```python
from build123d import *

# Parameters (mm, degrees)
ESTRUSIONE_ESTRUSIONE1_DEPTH      = 10
ESTRUSIONE_ESTRUSIONE1_DEPTH_BACK = 3
SCHIZZO1_W                        = 89
SCHIZZO1_H                        = 2
SCHIZZO2_W                        = 25
SCHIZZO2_H                        = 2
TAGLIO_ESTRUSIONE1_DEPTH          = 10
SCHIZZO3_W                        = 20
SCHIZZO3_H                        = 3
TAGLIO_ESTRUSIONE2_DEPTH          = 10
RACCORDO1_R                       = 8


with BuildPart() as part:
    # Schizzo1 → Estrusione-Estrusione1 (new, two sides: drawn at the far end of the back side and taken through both)
    with BuildSketch(Plane.XY.offset(-ESTRUSIONE_ESTRUSIONE1_DEPTH_BACK)):
        with Locations((0, 22.5)):
            Rectangle(SCHIZZO1_W, SCHIZZO1_H)
    extrude(amount=ESTRUSIONE_ESTRUSIONE1_DEPTH + ESTRUSIONE_ESTRUSIONE1_DEPTH_BACK)

    # Schizzo2 → Taglio-Estrusione1 (cut)
    with BuildSketch(Plane.XZ.offset(-21.5)):
        with Locations((-25, 6)):
            Rectangle(SCHIZZO2_W, SCHIZZO2_H)
        with Locations((25, 6)):
            Rectangle(SCHIZZO2_W, SCHIZZO2_H)
    extrude(amount=-TAGLIO_ESTRUSIONE1_DEPTH, mode=Mode.SUBTRACT)

    # Schizzo3 → Taglio-Estrusione2 (cut)
    with BuildSketch(Plane(origin=(0, 23.5, 0), x_dir=(1, 0, 0), z_dir=(0, 1, 0))):
        with Locations((0, 1.5)):
            Rectangle(SCHIZZO3_W, SCHIZZO3_H)
    extrude(amount=-TAGLIO_ESTRUSIONE2_DEPTH, mode=Mode.SUBTRACT)

    # Raccordo1
    raccordo1_edges = [part.edges().sort_by_distance(p)[0] for p in [
        (-44.5, 22.5, 10),
        (44.5, 22.5, 10),
    ]]
    fillet(raccordo1_edges, radius=RACCORDO1_R)


solid = part.part
```
Check sheet for the modelled part. Datum: model origin and axes. Units: mm. A direction names the side the tool comes from. Round coordinates to 2 decimals unless told otherwise and drop trailing zeros. Loops run counter-clockwise (first coordinate to the right, second up) from the corner with the lowest first, then second, coordinate; pieces in that order, holes last. Notation, with made-up numbers: (-10.5, 51.25) -> (41.5, 51.25) arc R25 ccw to (41.5, 63.25) -> close; hole circle Ø6 at (-3, 79). An arc over 180 degrees is marked (long way). Write item = value, one per line. Start each with the question number.
1) Release check for a two-part mould opening along X. For faces 4 (the flat face through (27, 23, -3)), 5 (the cylindrical face through (-42.219, 22.514, 7.594)), 6 (the flat face through (10, 23, -1)) record: released by +X, released by -X, zero draft, split by the parting line, or undercut.
2) Sectioned sample at C-C, the plane y = 22.15. Record the cut outline in (x, z), plus the area to 3 significant figures.
3) Sectioned sample at B-B, the plane z = -0.75. Record the cut outline in (x, y).
4) Gauge pin test, flat ends, axial feed: pin 1 Ø0.6 at (y, z) = (22.5, 6) entering from +X; pin 2 Ø1 at (y, z) = (22, 5.5) entering from -X; pin 3 Ø5 at (x, z) = (-18.5, 5.5) entering from -Y; pin 4 Ø1 at (y, z) = (22.5, 6.5) entering from -X. Record the tip position at first contact, or that the pin passes through.
5) Set-up check for faces 1 (the flat face through (0, 23, 0)), 2 (the flat face through (12.5, 22, 6)), 3 (the flat face through (-1, 23.5, 3)): record each of +Z, -Z, +X, -X, +Y, -Y from which the full face is reachable in a straight line by a thin tool's end or side.
6) Sectioned sample at A-A, the plane x = 19. Record the cut outline in (y, z), plus the area to 3 significant figures.
7) Sectioned sample at D-D, the plane x = 5. Record the cut outline in (y, z), plus the area to 3 significant figures.
8) Thickness scan on probe 1 along X at (y, z) = (21.7, -1.5); probe 2 along Z at (x, y) = (29, 22.4); probe 3 along X at (y, z) = (22, 6). Record the ranges inside material, lowest first.
Results are:
q1.face_4 = zero draft
q1.face_5 = released by -X
q1.face_6 = undercut
q2.outline = (-44.5, -3) -> (-10, -3) -> (-10, 0) -> (10, 0) -> (10, -3) -> (44.5, -3) -> (44.5, 2) arc R8 ccw to (36.5, 10) -> (-36.5, 10) arc R8 ccw to (-44.5, 2) -> close; hole (-37.5, 5) -> (-12.5, 5) -> (-12.5, 7) -> (-37.5, 7) -> close; hole (12.5, 5) -> (37.5, 5) -> (37.5, 7) -> (12.5, 7) -> close
q2.area = 970 mm^2
q3.outline = (-44.5, 21.5) -> (-10, 21.5) -> (-10, 23.5) -> (-44.5, 23.5) -> close; (10, 21.5) -> (44.5, 21.5) -> (44.5, 23.5) -> (10, 23.5) -> close
q4.pin_1 = 43.59
q4.pin_2 = -43.92
q4.pin_3 = 21.5
q4.pin_4 = -43.43
q5.face_1 = -Z, +Y, -Y
q5.face_2 = +Y, -Y
q5.face_3 = +Z, -Z, +X, -X, +Y
q6.outline = (21.5, -3) -> (23.5, -3) -> (23.5, 5) -> (21.5, 5) -> close; (21.5, 7) -> (23.5, 7) -> (23.5, 10) -> (21.5, 10) -> close
q6.area = 22.0 mm^2
q7.outline = (21.5, 0) -> (23.5, 0) -> (23.5, 10) -> (21.5, 10) -> close
q7.area = 20.0 mm^2
q8.probe_1 = -44.5 to -10, 10 to 44.5
q8.probe_2 = -3 to 5, 7 to 10
q8.probe_3 = -43.43 to -37.5, -12.5 to 12.5, 37.5 to 43.43
